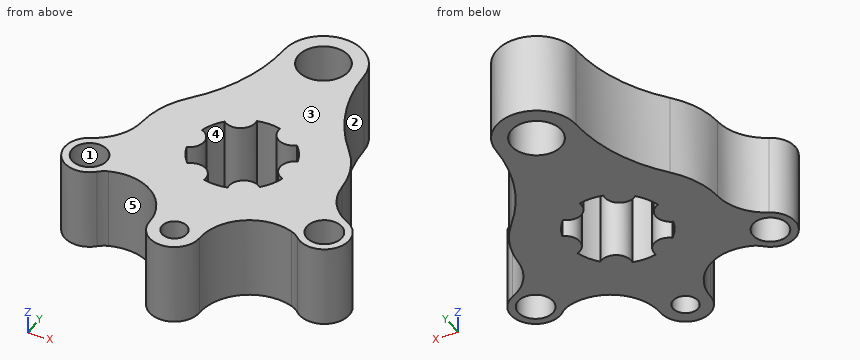
```python
from build123d import *

# Parameters (mm, degrees)
SKETCH1_R           = 7
SKETCH1_R_2         = 5
SKETCH1_R_3         = 10
BOSS_EXTRUDE1_DEPTH = 33


with BuildPart() as part:
    # Sketch1 → Boss-Extrude1 (new body)
    with BuildSketch(Plane.XY):
        with BuildLine():
            ThreePointArc((15.994033369, 60.436917155), (0, 76), (-15.994033369, 60.436917155))
            ThreePointArc((-15.994033369, 60.436917155), (-20.382321677, 38.833168081), (-31.840542672, 20))
            ThreePointArc((-31.840542672, 20), (-37.590888328, 10.684300366), (-39.97719521, 0))
            ThreePointArc((-39.97719521, 0), (-43.316807871, -10.045731282), (-51.316335778, -16.979509689))
            ThreePointArc((-51.316335778, -16.979509689), (-55.247302477, -31.655263199), (-40.141001052, -33.276959078))
            ThreePointArc((-40.141001052, -33.276959078), (-38.467197276, -32.003260227), (-36.564004207, -31.107836313))
            ThreePointArc((-36.564004207, -31.107836313), (-18.40862571, -33.701532524), (-10, -50))
            ThreePointArc((-10, -50), (0, -60), (10, -50))
            ThreePointArc((10, -50), (18.40862571, -33.701532524), (36.564004207, -31.107836313))
            ThreePointArc((36.564004207, -31.107836313), (38.467197276, -32.003260227), (40.141001052, -33.276959078))
            ThreePointArc((40.141001052, -33.276959078), (55.247302477, -31.655263199), (51.316335778, -16.979509689))
            ThreePointArc((51.316335778, -16.979509689), (43.316807871, -10.045731282), (39.97719521, 0))
            ThreePointArc((39.97719521, 0), (37.590888328, 10.684300366), (31.840542672, 20))
            ThreePointArc((31.840542672, 20), (20.382321677, 38.833168081), (15.994033369, 60.436917155))
        make_face()
        with Locations((-47, -26)):
            Circle(SKETCH1_R, mode=Mode.SUBTRACT)
        with Locations((0, -50)):
            Circle(SKETCH1_R_2, mode=Mode.SUBTRACT)
        with BuildLine():
            ThreePointArc((-14.486315543, 13.789367716), (-7.601024573, 13.16536075), (-4.698784972, 19.440201125))
            ThreePointArc((-4.698784972, 19.440201125), (0, 20), (4.698784972, 19.440201125))
            ThreePointArc((4.698784972, 19.440201125), (7.601024573, 13.16536075), (14.486315543, 13.789367716))
            ThreePointArc((14.486315543, 13.789367716), (17.320508076, 10), (19.185100515, 5.65083341))
            ThreePointArc((19.185100515, 5.65083341), (15.202049146, 0), (19.185100515, -5.65083341))
            ThreePointArc((19.185100515, -5.65083341), (17.320508076, -10), (14.486315543, -13.789367716))
            ThreePointArc((14.486315543, -13.789367716), (7.601024573, -13.16536075), (4.698784972, -19.440201125))
            ThreePointArc((4.698784972, -19.440201125), (0, -20), (-4.698784972, -19.440201125))
            ThreePointArc((-4.698784972, -19.440201125), (-7.601024573, -13.16536075), (-14.486315543, -13.789367716))
            ThreePointArc((-14.486315543, -13.789367716), (-17.320508076, -10), (-19.185100515, -5.65083341))
            ThreePointArc((-19.185100515, -5.65083341), (-15.202049146, 0), (-19.185100515, 5.65083341))
            ThreePointArc((-19.185100515, 5.65083341), (-17.320508076, 10), (-14.486315543, 13.789367716))
        make_face(mode=Mode.SUBTRACT)
        with Locations((47, -26)):
            Circle(SKETCH1_R, mode=Mode.SUBTRACT)
        with Locations((0, 60)):
            Circle(SKETCH1_R_3, mode=Mode.SUBTRACT)
    extrude(amount=BOSS_EXTRUDE1_DEPTH)


solid = part.part
```
Geometry check sheet. Reference: the model listing, model coordinates, mm. Face numbers are marked on the shaded views. A direction names the side the tool comes from. Round coordinates to 2 decimals unless told otherwise and drop trailing zeros. Loops run counter-clockwise (first coordinate to the right, second up) from the corner with the lowest first, then second, coordinate; pieces in that order, holes last. Notation, with made-up numbers: (11.5, 40.5) -> (20.5, 40.5) arc R16 ccw to (20.5, 66.5) -> close; hole circle Ø8 at (-10, -21.75). An arc over 180 degrees is marked (long way). Use a Markdown table: item, result.
(1) Sectioned sample at D-D (y = 54). Enter the section's corners in (x, z).
Calculated:
| item | result |
|---|---|
| outline | (-16.5, 0) -> (-8, 0) -> (-8, 33) -> (-16.5, 33) -> close; (8, 0) -> (16.5, 0) -> (16.5, 33) -> (8, 33) -> close |
(2) Sectioned sample at A-A (y = -26). Enter the section's corners in (x, z).
Calculated:
| item | result |
|---|---|
| outline | (-57, 0) -> (-54, 0) -> (-54, 33) -> (-57, 33) -> close; (-40, 0) -> (40, 0) -> (40, 33) -> (-40, 33) -> close; (54, 0) -> (57, 0) -> (57, 33) -> (54, 33) -> close |
(3) Sectioned sample at B-B (z = 20.5). Give the number of separate pieces and of enclosed holes in the cut face, then the cut area to 3 significant figures.
Calculated:
| item | result |
|---|---|
| separate pieces | 1 |
| enclosed holes | 5 |
| area | 5,690 mm² |
(4) Scan lines: probe 1 along X at (y, z) = (-25.5, 5); probe 2 along Y at (x, z) = (-4, 8.5); probe 3 along X at (y, z) = (-15.5, 11). Record each from-to range of solid material in increasing order.
Calculated:
| item | result |
|---|---|
| probe 1 | -56.99 to -53.98, -40.02 to 40.02, 53.98 to 56.99 |
| probe 2 | -59.17 to -53, -47 to -19.6, 19.6 to 50.83, 69.17 to 75.49 |
| probe 3 | -48.74 to -5.33, 5.33 to 48.74 |
(5) Sectioned sample at C-C (x = 0). Enter the section's corners in (y, z), then the cut area to 3 significant figures.
Calculated:
| item | result |
|---|---|
| outline | (-60, 0) -> (-55, 0) -> (-55, 33) -> (-60, 33) -> close; (-45, 0) -> (-20, 0) -> (-20, 33) -> (-45, 33) -> close; (20, 0) -> (50, 0) -> (50, 33) -> (20, 33) -> close; (70, 0) -> (76, 0) -> (76, 33) -> (70, 33) -> close |
| area | 2,180 mm² |
(6) Set-up check for the marked faces 4 and 5: record each of +Z, -Z, +X, -X, +Y, -Y from which the full face is reachable in a straight line by a thin tool's end or side.
Calculated:
| item | result |
|---|---|
| face 4 | +Z, -Z |
| face 5 | +Z, -Z, -Y |
(7) Mould release check, pull along X, two halves, no side actions. Record for the marked faces 1, 2 and 3: released by +X, released by -X, zero draft, split by the parting line, or undercut.
Calculated:
| item | result |
|---|---|
| face 1 | undercut |
| face 2 | released by +X |
| face 3 | zero draft |
(8) Go/stop test with flat-tipped pins: P1, Ø1.5, axis at y = 39, z = 19.5, coming from the +X side; P2, Ø1, axis at x = -36.5, z = 23.5, coming from the +Y side; P3, Ø1.5, axis at y = -44, z = 14, coming from the +X side; P4, Ø8.5, axis at x = -47, y = -26, coming from the -Z side. Record where each tip stops, or that it passes through.
Calculated:
| item | result |
|---|---|
| P1 | x = 20.61 |
| P2 | y = 14.04 |
| P3 | x = 11.17 |
| P4 | through |
